Autodesk Inventor part; units mm, degrees
ref_plane "YZ Plane" through (0, 0, 0) normal (1, 0, 0) x (0, 1, 0)
ref_plane "XZ Plane" through (0, 0, 0) normal (0, 1, 0) x (-1, 0, 0)
ref_plane "XY Plane" through (0, 0, 0) normal (0, 0, 1) x (1, 0, 0)
sketch "Skizze1" plane through (0, 0, 0) normal (0, 0, 1) x (1, 0, 0)
  circle A0 centre (0.0001, -0.0022) radius 3.9802
  circle A1 centre (-8.37, 7.9978) radius 1.4
  circle A2 centre (8.3745, -8.0022) radius 1.4
  line L0 (-9.5383, 7.2264) -> (-3.2198, -2.3418)
  line L1 (-7.6522, 9.1998) -> (1.8915, 3.4999)
  line L2 (9.5428, -7.2307) -> (3.3215, 2.191)
  line L3 (-1.8517, -3.5253) -> (7.6567, -9.2041)
  point P0 (0, 0)
extrude "Extrusion1" add sketch "Skizze1" along normal blind 4
sketch "Skizze2" plane through (0, 0, 4) normal (0, 0, 1) x (1, 0, 0)
  arc A0 (-7.6522, 9.1998) -> (-9.5383, 7.2264) centre (-8.37, 7.9978) ccw
  line L0 (-9.5383, 7.2264) -> (-3.2198, -2.3418)
  arc A1 (-3.2198, -2.3418) -> (-1.8517, -3.5253) centre (0.0001, -0.0022) ccw
  line L1 (-1.8517, -3.5253) -> (7.6567, -9.2041)
  arc A2 (7.6567, -9.2041) -> (9.5428, -7.2307) centre (8.3745, -8.0022) ccw
  line L2 (9.5428, -7.2307) -> (3.3215, 2.191)
  arc A3 (3.3215, 2.191) -> (1.8915, 3.4999) centre (0.0001, -0.0022) ccw
  line L3 (1.8915, 3.4999) -> (-7.6522, 9.1998)
  arc A4 (-6.6267, 10.9169) -> (-11.2072, 6.1243) centre (-8.37, 7.9978) ccw
  line L4 (-11.2072, 6.1243) -> (-4.8666, -3.4774)
  arc A5 (-4.8666, -3.4774) -> (-2.8352, -5.2674) centre (0.0001, -0.0022) ccw
  line L5 (-2.8352, -5.2674) -> (6.6312, -10.9212)
  arc A6 (6.6312, -10.9212) -> (11.2118, -6.1287) centre (8.3745, -8.0022) ccw
  line L6 (11.2118, -6.1287) -> (4.9905, 3.2931)
  arc A7 (4.9905, 3.2931) -> (2.8837, 5.2369) centre (0.0001, -0.0022) ccw
  line L7 (2.8837, 5.2369) -> (-6.6267, 10.9169)
  point P0 (0, 0)
  dimension "d2" = 2
extrude "Extrusion2" add sketch "Skizze2" against normal up to surface (4 mm away)
sketch "Skizze3" plane through (0, 0, 4) normal (0, 0, 1) x (1, 0, 0)
  circle A0 centre (0.0001, -0.0022) radius 3.9802
  circle A1 centre (-8.37, 7.9978) radius 1.4
  circle A2 centre (8.3745, -8.0022) radius 1.4
  circle A3 centre (0.0001, -0.0022) radius 3.35
  point P0 (0, 0)
  dimension "d5" = 6.7
extrude "Extrusion3" cut sketch "Skizze3" against normal through all contours A1 | A2 | A3
sketch "Skizze4" plane through (0, 0, 4) normal (0, 0, 1) x (1, 0, 0)
  circle A0 centre (-8.37, 7.9978) radius 1.4
  circle A1 centre (8.3745, -8.0022) radius 1.4
  point P0 (0, 0)
hole "Bohrung1" at (-8.37, 7.9978, 4) at (8.3745, -8.0022, 4) direction (0, 0, -1) diameter 2.8 end through all counterbore diameter 6 counterbore depth 2.5
properties part number "IM_Lensholder"
Verification items for the finished model (mm, model axes). A direction names the side the tool comes from. Coordinates: 2 decimals unless noted, no trailing zeros. Write each loop counter-clockwise with the first axis right and the second up, starting at its lowest first coordinate (ties: lowest second). Pieces come first, ordered by that corner, then holes. Notation, with made-up numbers: M 62.25,26.5 L 102.25,26.5 A31 ccw 102.25,50.5 Z; hole C 33,3 d5. An arc over 180 degrees is marked long. Answer as a JSON object with one key per item and string values. Group by question number.
(1) Cross-section at B-B, the plane x = -2.5. Record the cut outline in (y, z).
(2) Gauge pin test, flat ends, axial feed: pin 1 (3.5 mm diameter, centred on x = 8.37, y = -8, fed in from +Z); pin 2 (5.5 mm diameter, centred on x = 0, y = 0, fed in from -Z); pin 3 (2 mm diameter, centred on y = 5.5, z = 1, fed in from +X). Record the tip position at first contact, or that the pin passes through.
(3) Material ranges on line 1 (X direction, y = -0.75, z = 2.75); line 2 (Y direction, x = 0, z = 0.6); line 3 (Y direction, x = -8.37, z = 1.2), recorded low to high.
(4) Release check for a two-part mould opening along Y. For faces 1 (the face through (2, 3, 0)), 2 (the face through (1.55, -2.97, 2.03)), 3 (the face through (8.14, -1.48, 2.03)) record: +Y half, -Y half, draft (parallel to the pull), parting line (faces both ways), or undercut.
(5) Cross-section at D-D, the plane z = 2.3. Record the cut outline in (x, y).
(6) Cross-section at C-C, the plane z = 0.8. Record the cut outline in (x, y), and give its area (3 significant figures).
(7) Cross-section at A-A, the plane y = 1. Record the cut outline in (x, z).
(8) Tool access check on faces 4 (the face through (7.473, -10.864, 2.732)), 5 (the face through (-10.783, 10.393, 2.028)). Record the directions out of +Z, -Z, +X, -X, +Y, -Y that give a thin tool (end or side, any length) a straight path to the whole face; none if there is none.
Reply:
{
 "1": {"outline": "M -5.47,0 L -2.23,0 L -2.23,4 L -5.47,4 Z; M 2.23,0 L 8.45,0 L 8.45,4 L 2.23,4 Z"},
 "2": {"pin 1": "z = 1.5", "pin 2": "through", "pin 3": "x = 3.94"},
 "3": {"line 1": "-6.67 to -3.27, 3.27 to 7.66", "line 2": "-6.96 to -3.35, 3.35 to 6.96", "line 3": "1.83 to 6.6, 9.4 to 11.4"},
 "4": {"face 1": "draft", "face 2": "undercut", "face 3": "+Y half"},
 "5": {"outline": "M -11.21,6.12 L -4.87,-3.48 A5.98 ccw -2.84,-5.27 L 6.63,-10.92 A3.4 ccw 11.21,-6.13 L 4.99,3.29 A5.98 ccw 2.88,5.24 L -6.63,10.92 A3.4 ccw Z; hole C -8.37,8 d6; hole C 0,0 d6.7; hole C 8.37,-8 d6"},
 "6": {"outline": "M -11.21,6.12 L -4.87,-3.48 A5.98 ccw -2.84,-5.27 L 6.63,-10.92 A3.4 ccw 11.21,-6.13 L 4.99,3.29 A5.98 ccw 2.88,5.24 L -6.63,10.92 A3.4 ccw Z; hole C -8.37,8 d2.8; hole C 0,0 d6.7; hole C 8.37,-8 d2.8", "area": "211 mm²"},
 "7": {"outline": "M -7.82,0 L -3.2,0 L -3.2,4 L -7.82,4 Z; M 3.2,0 L 6.5,0 L 6.5,4 L 3.2,4 Z"},
 "8": {"face 4": "+Z", "face 5": "+Z, -Z"}
}
